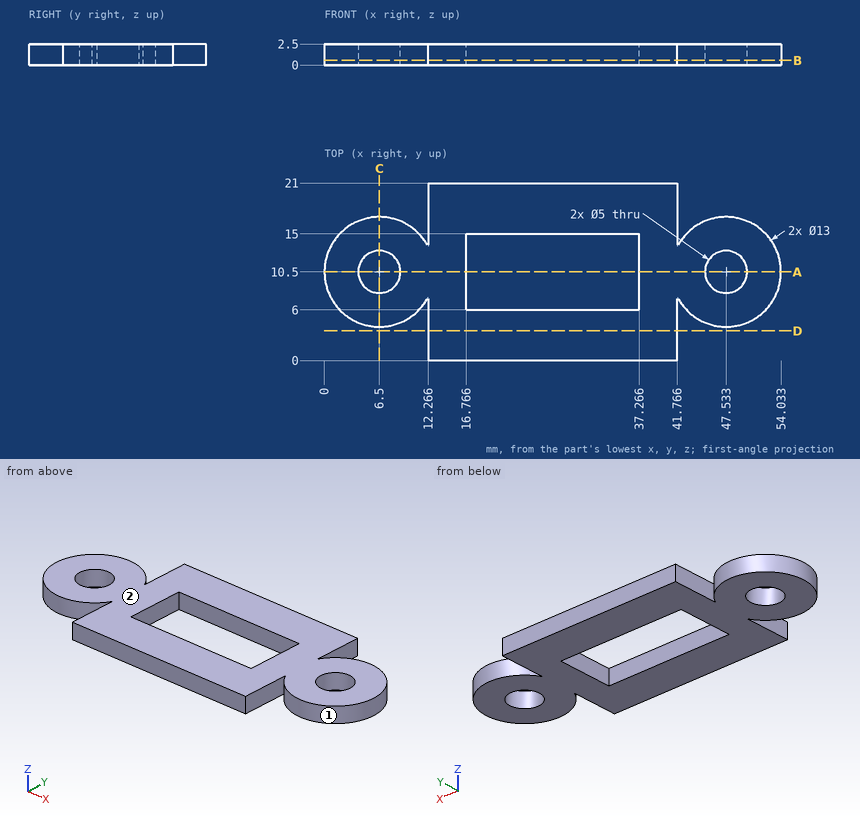
Source: three-view drawing plus pictorial views. Frame: mm from the lowest corner of the part. Give positions to 0.01 mm unless a question says otherwise; leave off trailing zeros. Loops run counter-clockwise (first coordinate to the right, second up) from the corner with the lowest first, then second, coordinate; pieces in that order, holes last. Notation, with made-up numbers: M -33,59.25 L 17,59.25 A32 cw 17,96.25 Z; hole C 84,-23.75 d3. An arc over 180 degrees is marked long. Put each result on its own line as item: value.
Q1. Section A-A (y = 10.5). Return the cut outline in (x, z).
Response values:
outline: M 0,0 L 4,0 L 4,2.5 L 0,2.5 Z; M 9,0 L 16.77,0 L 16.77,2.5 L 9,2.5 Z; M 37.27,0 L 45.03,0 L 45.03,2.5 L 37.27,2.5 Z; M 50.03,0 L 54.03,0 L 54.03,2.5 L 50.03,2.5 Z
Q2. Section D-D (y = 3.5). Return the cut outline in (x, z).
Response values:
outline: M 12.27,0 L 41.77,0 L 41.77,2.5 L 12.27,2.5 Z
Q3. Pin query (flat end, axial travel): P1, Ø1.2, axis at y = 2.5, z = 1, coming from the +X side; P2, Ø0.8, axis at y = 4.5, z = 2, coming from the -X side; P3, Ø1, axis at y = 4.5, z = 0.5, coming from the +X side (1 decimal). Return the tip coordinate at first contact, or that it passes through.
Response values:
P1: stops at x = 41.77
P2: stops at x = 3.2
P3: stops at x = 51
Q4. Line query: probe 1 along Y at (x, z) = (17, 1.9); probe 2 along Y at (x, z) = (6.5, 1.6); probe 3 along X at (y, z) = (9, 0.7) (1 decimal). Output: solid intervals per line, ascending. Write a range as [from, to].
Response values:
probe 1: y = [0, 6], [15, 21]
probe 2: y = [4, 8], [13, 17]
probe 3: x = [0.2, 4.5], [8.5, 16.8], [37.3, 45.5], [49.5, 53.9]
Q5. Section B-B (z = 0.55). Return the cut outline in (x, y).
Response values:
outline: M 12.27,0 L 41.77,0 L 41.77,7.5 A6.5 ccw long 41.77,13.5 L 41.77,21 L 12.27,21 L 12.27,13.5 A6.5 ccw long 12.27,7.5 Z; hole C 6.5,10.5 d5; hole M 16.77,6 L 37.27,6 L 37.27,15 L 16.77,15 Z; hole C 47.53,10.5 d5
Q6. Section C-C (x = 6.5). Return the cut outline in (y, z).
Response values:
outline: M 4,0 L 8,0 L 8,2.5 L 4,2.5 Z; M 13,0 L 17,0 L 17,2.5 L 13,2.5 Z
Q7. Mould query, pull axis X, two halves, no side actions, for the marked faces 1 and 2. Classes: released by +X, released by -X, zero draft, split by the parting line, or undercut.
Response values:
face 1: undercut
face 2: zero draft
